```python
from build123d import *

# Parameters (mm, degrees)
SKETCH_R        = 25
PAD_DEPTH       = 2
SKETCH001_R     = 13.05
POCKET_DEPTH    = 5
SKETCH002_W     = 5
SKETCH002_H     = 2.5
PAD001_DEPTH    = 13
SKETCH003_R     = 1.25
POCKET001_DEPTH = 5
SKETCH004_W     = 5
SKETCH004_H     = 2.5
PAD002_DEPTH    = 5
SKETCH005_W     = 0.35
SKETCH005_H     = 10
PAD003_DEPTH    = 0.3


with BuildPart() as part:
    # Sketch → Pad (new body)
    with BuildSketch(Plane.XY):
        Circle(SKETCH_R)
    extrude(amount=PAD_DEPTH)

    # Sketch001 → Pocket (cut)
    with BuildSketch(Plane.XY.offset(2)):
        Circle(SKETCH001_R)
    extrude(amount=-POCKET_DEPTH, mode=Mode.SUBTRACT)

    # Sketch002 → Pad001 (new body)
    with BuildSketch(Plane.XY.offset(2)):
        with Locations((-18, -7.25)):
            Rectangle(SKETCH002_W, SKETCH002_H)
        with Locations((18, -7.25)):
            Rectangle(SKETCH002_W, SKETCH002_H)
    extrude(amount=PAD001_DEPTH)

    # Sketch003 → Pocket001 (cut)
    with BuildSketch(Plane.XZ.offset(8.5)):
        with Locations((-18, 12)):
            Circle(SKETCH003_R)
        with Locations((18, 12)):
            Circle(SKETCH003_R)
    extrude(amount=-POCKET001_DEPTH, mode=Mode.SUBTRACT)

    # Sketch004 → Pad002 (new body)
    with BuildSketch(Plane.XY.offset(2)):
        with Locations((-18, -4.75)):
            Rectangle(SKETCH004_W, SKETCH004_H)
        with Locations((18, -4.75)):
            Rectangle(SKETCH004_W, SKETCH004_H)
    extrude(amount=PAD002_DEPTH)

    # Sketch005 → Pad003 (new body)
    with BuildSketch(Plane.XY.offset(2)):
        with Locations((0, -19)):
            Rectangle(SKETCH005_W, SKETCH005_H)
    extrude(amount=PAD003_DEPTH)


solid = part.part
```
Model file for the job. Use its own axes, mm. A direction names the side the tool comes from. Coordinates: 2 decimals unless noted, no trailing zeros. Loops run counter-clockwise (first coordinate to the right, second up) from the corner with the lowest first, then second, coordinate; pieces in that order, holes last. Notation, with made-up numbers: (88, 80) -> (136, 80) arc R21 ccw to (136, 104) -> close; hole circle Ø11 at (34, -16). An arc over 180 degrees is marked (long way). Answer as a JSON object with one key per item and string values.
Q1. Flat gauge pins, fed straight in: P1, Ø5.5, axis at y = -5.5, z = 5.5, coming from the +X side; P2, Ø12, axis at x = -15, y = 19.5, coming from the +Z side; P3, Ø6, axis at x = 10.5, z = 2.5, coming from the +Y side; P4, Ø5, axis at x = 11.5, y = 17, coming from the -Z side. Where does each tip first touch, or does it go through?
Report:
{"P1": "stops at x = 20.5", "P2": "stops at z = 2", "P3": "stops at y = 23.84", "P4": "stops at z = 0"}
Q2. Cut at D-D (y = -5). List the corners of the cut face in (x, z), and give its area (3 significant figures).
Report:
{"outline": "(-24.49, 0) -> (-12.05, 0) -> (-12.05, 2) -> (-15.5, 2) -> (-15.5, 7) -> (-20.5, 7) -> (-20.5, 2) -> (-24.49, 2) -> close; (12.05, 0) -> (24.49, 0) -> (24.49, 2) -> (20.5, 2) -> (20.5, 7) -> (15.5, 7) -> (15.5, 2) -> (12.05, 2) -> close", "area": "99.8 mm2"}
Q3. Pull direction Y, two halves, no side cores. Call faces 1 (the flat face through (18, -7, 15)), 2 (the flat face through (-18, -3.5, 4)), 3 (the cylindrical face through (-9.62, 8.82, 1.01)): released by +Y, released by -Y, zero draft, split by the parting line, or undercut.
Report:
{"face 1": "zero draft", "face 2": "released by +Y", "face 3": "undercut"}
Q4. Cut at C-C (x = 18). List the corners of the cut face in (y, z), and give its area (3 significant figures).
Report:
{"outline": "(-17.35, 0) -> (17.35, 0) -> (17.35, 2) -> (-3.5, 2) -> (-3.5, 7) -> (-6, 7) -> (-6, 10.75) -> (-8.5, 10.75) -> (-8.5, 2) -> (-17.35, 2) -> close; (-8.5, 13.25) -> (-6, 13.25) -> (-6, 15) -> (-8.5, 15) -> close", "area": "108 mm2"}
Q5. Cut at A-A (z = 3). List the corners of the cut face in (x, y), and give its area (3 significant figures).
Report:
{"outline": "(-20.5, -8.5) -> (-15.5, -8.5) -> (-15.5, -3.5) -> (-20.5, -3.5) -> close; (15.5, -8.5) -> (20.5, -8.5) -> (20.5, -3.5) -> (15.5, -3.5) -> close", "area": "50.0 mm2"}
Q6. Cut at B-B (y = 0). List the corners of the cut face in (x, z), and give its area (3 significant figures).
Report:
{"outline": "(-25, 0) -> (-13.05, 0) -> (-13.05, 2) -> (-25, 2) -> close; (13.05, 0) -> (25, 0) -> (25, 2) -> (13.05, 2) -> close", "area": "47.8 mm2"}
Q7. Probe probe 1 along Y at (x, z) = (0, 0.6); probe 2 along Z at (x, y) = (-18, -7.55); probe 3 along Z at (x, y) = (-17.5, 7). List the from-to ranges inside material, lowest first.
Report:
{"probe 1": "y = -25 to -13.05, 13.05 to 25", "probe 2": "z = 0 to 10.75, 13.25 to 15", "probe 3": "z = 0 to 2"}
Q8. 3-axis set-ups, long thin cutter, end or side, ignore diameter. For faces 4 (the flat face through (15.5, -7, 7)), 5 (the flat face through (18, -5, 7)), 6 (the flat face through (-20.5, -7, 7)): which of +Z, -Z, +X, -X, +Y, -Y reach the whole face in a straight line?
Report:
{"face 4": "+Z, +Y, -Y", "face 5": "+Z, +X, -X, +Y", "face 6": "+Z, -X, +Y, -Y"}
